Design review of the part built by this model. Coordinates are the model's own, in mm. Face numbers are marked on the shaded views. A direction names the side the tool comes from. Round coordinates to 2 decimals unless told otherwise and drop trailing zeros. Order: outer loops, then holes, each group sorted by start corner. A loop starts at its lowest first (then second) coordinate and runs counter-clockwise, first axis right, second up.
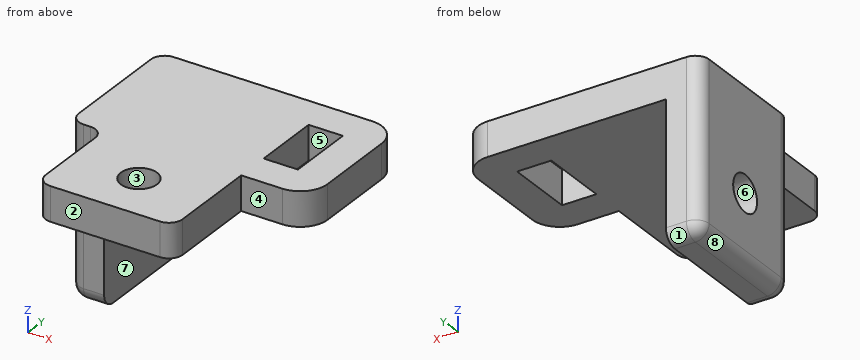
from build123d import *

# Parameters (mm, degrees)
CROQUIS1_W              = 5
CROQUIS1_H              = 10
SALIENTE_EXTRUIR1_DEPTH = 5
CROQUIS2_W              = 5
CROQUIS2_H              = 20
SALIENTE_EXTRUIR3_DEPTH = 25
CROQUIS3_R              = 2.65
CORTAR_EXTRUIR1_DEPTH   = 42.533119315
CROQUIS4_W              = 20
CROQUIS4_H              = 15
CROQUIS4_R              = 2.65
SALIENTE_EXTRUIR4_DEPTH = 5
REDONDEO1_R             = 2
REDONDEO2_R             = 2
REDONDEO3_R             = 2
REDONDEO4_R             = 2


with BuildPart() as part:
    # Croquis1 → Saliente-Extruir1 (new body)
    with BuildSketch(Plane.XY):
        with BuildLine():
            Line((-15, -10), (11, -10))
            ThreePointArc((11, -10), (13.828427125, -8.828427125), (15, -6))
            Line((15, -6), (15, 6))
            ThreePointArc((15, 6), (13.828427125, 8.828427125), (11, 10))
            Line((11, 10), (-15, 10))
            Line((-15, 10), (-15, -10))
        make_face()
        with Locations((7.5, 0)):
            Rectangle(CROQUIS1_W, CROQUIS1_H, mode=Mode.SUBTRACT)
    extrude(amount=SALIENTE_EXTRUIR1_DEPTH)

    # Croquis2 → Saliente-Extruir3 (add)
    with BuildSketch(Plane.XY.offset(5)):
        with Locations((-17.5, 0)):
            Rectangle(CROQUIS2_W, CROQUIS2_H)
    extrude(amount=-SALIENTE_EXTRUIR3_DEPTH)

    # Croquis3 → Cortar-Extruir1 (cut, through all)
    with BuildSketch(Plane.ZY.offset(20)):
        with Locations(Location((-10, 0, 0), (0, 0, 270))):
            Circle(CROQUIS3_R)
    extrude(amount=-CORTAR_EXTRUIR1_DEPTH, mode=Mode.SUBTRACT)

    # Croquis4 → Saliente-Extruir4 (add)
    with BuildSketch(Plane.XY.offset(5)):
        with Locations((-5, -17.5)):
            Rectangle(CROQUIS4_W, CROQUIS4_H)
        with Locations((-5, -17.5)):
            Circle(CROQUIS4_R, mode=Mode.SUBTRACT)
    extrude(amount=-SALIENTE_EXTRUIR4_DEPTH)

    # Redondeo1
    redondeo1_edges = [part.edges().sort_by_distance(p)[0] for p in [
        (-15, -10, 2.5),
    ]]
    fillet(redondeo1_edges, radius=REDONDEO1_R)

    # Redondeo2
    redondeo2_edges = [part.edges().sort_by_distance(p)[0] for p in [
        (5, -25, 2.5),
        (-15, -25, 2.5),
    ]]
    fillet(redondeo2_edges, radius=REDONDEO2_R)

    # Redondeo3
    redondeo3_edges = [part.edges().sort_by_distance(p)[0] for p in [
        (-17.5, -10, -20),
        (-17.5, 10, -20),
    ]]
    fillet(redondeo3_edges, radius=REDONDEO3_R)

    # Redondeo4
    redondeo4_edges = [part.edges().sort_by_distance(p)[0] for p in [
        (-20, 10, -6.5),
        (-20, 0, -20),
        (-20, -10, -6.5),
        (-20, -9.414213562, -19.414213562),
        (-20, 9.414213562, -19.414213562),
    ]]
    fillet(redondeo4_edges, radius=REDONDEO4_R)


solid = part.part
1) To check wall thickness, follow line 1 along Y through (x, z) = (-5, 3.5); line 2 along Z through (x, y) = (-16, 0); line 3 along Z through (x, y) = (-6, -12). State the ranges of each line that lie inside material, in increasing order.
Results:
line 1: y = -25 to -20.15, -14.85 to 10
line 2: z = -20 to -12.65, -7.35 to 5
line 3: z = 0 to 5
2) Clearance check with flat-ended pins moving along their axes: P1, Ø0.9, axis at x = -17, z = -2.5, coming from the -Y side; P2, Ø8, axis at x = -4, y = -0.5, coming from the -Z side; P3, Ø2, axis at y = 2, z = -12, coming from the +X side. State where each tip first meets the part, or that it passes through.
Results:
P1: stops at y = -10
P2: stops at z = 0
P3: stops at x = -15
3) Take a section at C-C on y = -17.5. Give the boundary of the cut face in (x, z), plus the area to 3 significant figures.
Results:
outline: (-15, 0) - (-7.65, 0) - (-7.65, 5) - (-15, 5) - close; (-2.35, 0) - (5, 0) - (5, 5) - (-2.35, 5) - close
area: 73.5 mm2
4) The part is to be moulded in two halves that separate along Y. For the marked faces 1, 2 and 3, say which applies: released by +Y, released by -Y, zero draft, split by the parting line, or undercut.
Results:
face 1: released by +Y
face 2: released by -Y
face 3: undercut
5) Take a section at D-D on y = 0. Give the boundary of the cut face in (x, z), plus the area to 3 significant figures.
Results:
outline: (-20, -18) arc R2 ccw to (-18, -20) - (-15, -20) - (-15, -12.65) - (-20, -12.65) - close; (-20, -7.35) - (-15, -7.35) - (-15, 0) - (5, 0) - (5, 5) - (-20, 5) - close; (10, 0) - (15, 0) - (15, 5) - (10, 5) - close
area: 223 mm2
6) Take a section at A-A on z = -10. Give the boundary of the cut face in (x, y).
Results:
outline: (-20, -8) arc R2 ccw to (-18, -10) - (-15, -10) - (-15, -2.65) - (-20, -2.65) - close; (-20, 2.65) - (-15, 2.65) - (-15, 10) - (-18, 10) arc R2 ccw to (-20, 8) - close
7) For the marked faces 4, 5, 6, 7 and 8, list the 3-axis set-ups (+Z, -Z, +X, -X, +Y, -Y) from which the entire face can be reached by the end or side of a thin tool; tool diameter is ignored.
Results:
face 4: +Z, -Z, +X, -Y
face 5: +Z, -Z
face 6: +X, -X
face 7: -Z, +X, +Y, -Y
face 8: -Z, -X, +Y, -Y
8) Take a section at B-B on x = -5. Give the boundary of the cut face in (y, z).
Results:
outline: (-25, 0) - (-20.15, 0) - (-20.15, 5) - (-25, 5) - close; (-14.85, 0) - (10, 0) - (10, 5) - (-14.85, 5) - close
